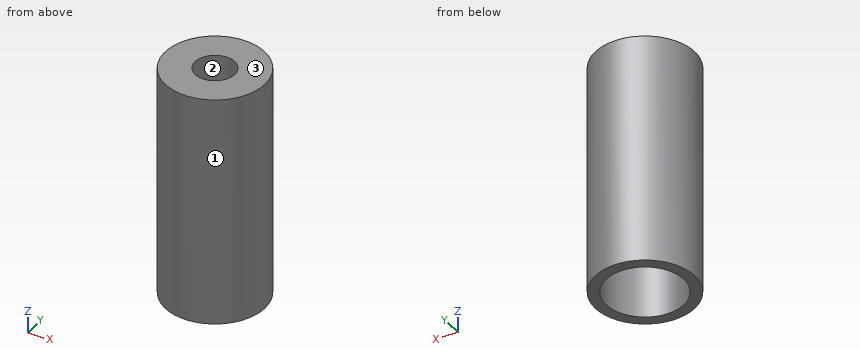
from build123d import *

# Parameters (mm, degrees)
F0_R     = 4.15
F0_R_2   = 3.25
F1_DEPTH = 6.3
F2_R     = 4.15
F3_DEPTH = 1
F4_R     = 1.65
F5_DEPTH = 1
F6_R     = 4.15
F6_R_2   = 1.65
F7_DEPTH = 12


with BuildPart() as f1:
    # F0 (on Top) → F1 (new body)
    with BuildSketch(Plane.XY):
        Circle(F0_R)
        Circle(F0_R_2, mode=Mode.SUBTRACT)
    extrude(amount=F1_DEPTH)

    # F2 (on face) → F3 (join)
    with BuildSketch(Plane.XY.offset(6.3)):
        Circle(F2_R)
    extrude(amount=F3_DEPTH)

    # F4 (on face) → F5 (cut, through all)
    with BuildSketch(Plane.XY.offset(7.3)):
        Circle(F4_R)
    extrude(amount=-F5_DEPTH, mode=Mode.SUBTRACT)

    # F6 (on face) → F7 (join)
    with BuildSketch(Plane.XY.offset(7.3)):
        Circle(F6_R)
        Circle(F6_R_2, mode=Mode.SUBTRACT)
    extrude(amount=F7_DEPTH)


solid = f1.part
Work out the finished part from the listing and answer in its coordinate system (mm). Face numbers are marked on the shaded views. Give positions to 0.01 mm unless a question says otherwise; leave off trailing zeros. Order: outer loops, then holes, each group sorted by start corner. A loop starts at its lowest first (then second) coordinate and runs counter-clockwise, first axis right, second up. Notation, with made-up numbers: M 38,-12.5 L 54,-12.5 A17 cw 54,18.5 Z; hole C 24,32.5 d3. An arc over 180 degrees is marked long. Return JSON: item names as keys, results as strings.
Q1. Each of these flat-tipped pins is pushed along its axis until it touches: pin 1 (3 mm diameter, centred on x = 0.5, y = 1, fed in from -Z); pin 2 (2 mm diameter, centred on y = -3, z = 7, fed in from -X). Where does it stop, or does it pass through?
Answer below:
{"pin 1": "stops at z = 6.3", "pin 2": "stops at x = -3.64"}
Q2. Find section C-C, the plane z = 3.75. Write down the section's boundary in (x, y), and give its area (3 significant figures).
Answer below:
{"outline": "C 0,0 d8.3; hole C 0,0 d6.5", "area": "20.9 mm^2"}
Q3. Find section A-A, the plane x = 0. Write down the section's boundary in (y, z).
Answer below:
{"outline": "M -4.15,0 L -3.25,0 L -3.25,6.3 L -1.65,6.3 L -1.65,19.3 L -4.15,19.3 Z; M 1.65,6.3 L 3.25,6.3 L 3.25,0 L 4.15,0 L 4.15,19.3 L 1.65,19.3 Z"}
Q4. The mould has two halves that part along Y. Classify the marked faces 1, 2 and 3: pulls with the +Y half, pulls with the -Y half, needs draft (parallel to the pull), parting line crosses it, or undercut.
Answer below:
{"face 1": "parting line crosses it", "face 2": "undercut", "face 3": "needs draft"}
Q5. Find the intervals of material crossed by line 1 along Y through (x, z) = (0, 4); line 2 along Z through (x, y) = (-2, 1.5); line 3 along Y through (x, z) = (0, 14.5), in increasing order. Write a range as [from, to].
Answer below:
{"line 1": "y = [-4.15, -3.25], [3.25, 4.15]", "line 2": "z = [6.3, 19.3]", "line 3": "y = [-4.15, -1.65], [1.65, 4.15]"}
Q6. Find section D-D, the plane y = -2.25. Write down the section's boundary in (x, z).
Answer below:
{"outline": "M -3.49,0 L -2.35,0 L -2.35,6.3 L 2.35,6.3 L 2.35,0 L 3.49,0 L 3.49,19.3 L -3.49,19.3 Z"}
